Design review of the part built by this model. Coordinates are the model's own, in mm. Face numbers are marked on the shaded views. A direction names the side the tool comes from. Round coordinates to 2 decimals unless told otherwise and drop trailing zeros. Loops run counter-clockwise (first coordinate to the right, second up) from the corner with the lowest first, then second, coordinate; pieces in that order, holes last. Notation, with made-up numbers: M 33,-21.5 L 42,-21.5 A20 ccw 42,15.5 Z; hole C 13.25,68.25 d3. An arc over 180 degrees is marked long. One line per item, written item: value. Start each with the question number.
Item 1: We need section D-D (z = -2.75). Write out the cut boundary in (x, y), then the cut area to 3 significant figures.
Item 2: We need section C-C (x = 4). Write out the cut boundary in (y, z), then the cut area to 3 significant figures.
Item 3: We need section A-A (y = 0). Write out the cut boundary in (x, z), then the cut area to 3 significant figures.
Item 4: Clearance check with flat-ended pins moving along their axes: pin 1 (3 mm diameter, centred on x = 32.5, z = 3.5, fed in from +Y); pin 2 (1 mm diameter, centred on x = 35, z = 1.5, fed in from -Y); pin 3 (2.5 mm diameter, centred on x = 4, y = 0, fed in from -Z). State where each tip first meets the part, or that it passes through.
Item 5: For the marked faces 1 and 2, list the 3-axis set-ups (+Z, -Z, +X, -X, +Y, -Y) from which the entire face can be reached by the end or side of a thin tool; tool diameter is ignored.
Item 6: For line 1 along X through (y, z) = (0, 1.75); line 2 along Y through (x, z) = (4, 0.5); line 3 along Y through (x, z) = (4, -1), list the stretches that pass through material, from the lowest coordinate up.
Item 7: We need section B-B (z = 0). Write out the cut boundary in (x, y), then the cut area to 3 significant figures.
from build123d import *

# Parameters (mm, degrees)
SKETCH1_R               = 3.5
BOSS_EXTRUDE1_DEPTH     = 60
SKETCH2_R               = 6
BOSS_EXTRUDE2_DEPTH     = 3
SKETCH3_R               = 1.5
CUT_EXTRUDE1_DEPTH      = 7
CUT_EXTRUDE1_DEPTH_BACK = 7


with BuildPart() as part:
    # Sketch1 → Boss-Extrude1 (new body)
    with BuildSketch(Plane(origin=(0, 0, 0), x_dir=(0, 0, -1), z_dir=(1, 0, 0))):
        Circle(SKETCH1_R)
    extrude(amount=BOSS_EXTRUDE1_DEPTH)

    # Sketch2 → Boss-Extrude2 (add)
    with BuildSketch(Plane(origin=(60, 0, 0), x_dir=(0, 0, -1), z_dir=(1, 0, 0))):
        Circle(SKETCH2_R)
    extrude(amount=BOSS_EXTRUDE2_DEPTH)

    # Sketch3 → Cut-Extrude1 (cut, two sides)
    with BuildSketch(Plane.XY) as cut_extrude1_sk:
        with Locations((4, 0)):
            Circle(SKETCH3_R)
    extrude(amount=CUT_EXTRUDE1_DEPTH, mode=Mode.SUBTRACT)
    extrude(cut_extrude1_sk.sketch, amount=-CUT_EXTRUDE1_DEPTH_BACK, mode=Mode.SUBTRACT)


solid = part.part
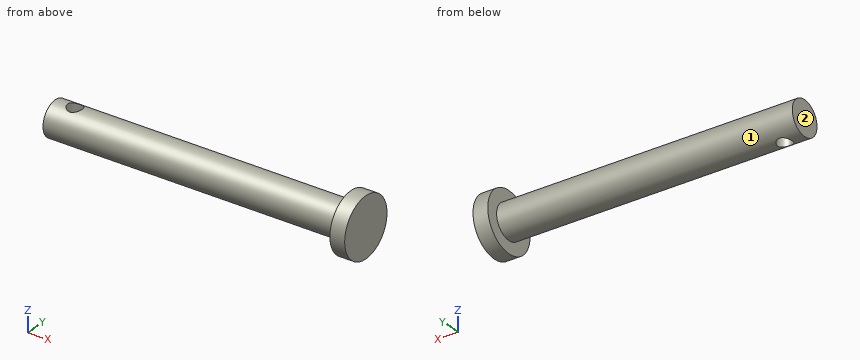
A:
1. outline: M 0,-2.17 L 60,-2.17 L 60,-5.33 L 63,-5.33 L 63,5.33 L 60,5.33 L 60,2.17 L 0,2.17 Z; hole C 4,0 d3
1. area: 285 mm2
2. outline: M -1.5,-3.16 L -1.5,3.16 A3.5 ccw Z; M 1.5,-3.16 A3.5 ccw 1.5,3.16 Z
2. area: 18.1 mm2
3. outline: M 0,-3.5 L 2.5,-3.5 L 2.5,3.5 L 0,3.5 Z; M 5.5,-3.5 L 60,-3.5 L 60,-6 L 63,-6 L 63,6 L 60,6 L 60,3.5 L 5.5,3.5 Z
3. area: 435 mm2
4. pin 1: y = 2.87
4. pin 2: y = -3.35
4. pin 3: through
5. face 1: -X
5. face 2: +Z, -Z, -X, +Y, -Y
6. line 1: 0 to 2.5, 5.5 to 63
6. line 2: -3.46 to -1.5, 1.5 to 3.46
6. line 3: -3.35 to -1.5, 1.5 to 3.35
7. outline: M 0,-3.5 L 60,-3.5 L 60,-6 L 63,-6 L 63,6 L 60,6 L 60,3.5 L 0,3.5 Z; hole C 4,0 d3
7. area: 449 mm2
